Model file for the job. Use its own axes, mm. Face numbers are marked on the shaded views. A direction names the side the tool comes from. Coordinates: 2 decimals unless noted, no trailing zeros. Write each loop counter-clockwise with the first axis right and the second up, starting at its lowest first coordinate (ties: lowest second). Pieces come first, ordered by that corner, then holes. Notation, with made-up numbers: (45.25, 23.25) - (97.25, 23.25) arc R19 cw to (97.25, 55.25) - close; hole circle Ø11 at (1.25, 53.25). An arc over 180 degrees is marked (long way). Put each result on its own line as item: value. Start each with the question number.
1. Saw through at D-D, the plane z = -13. Write the cut outline in (x, y), plus the area to 3 significant figures.
2. Drop flat-ended pins along their axis: P1, Ø5, axis at y = -3.5, z = -8, coming from the -X side; P2, Ø2, axis at y = 1.5, z = -7, coming from the -X side; P3, Ø1, axis at y = 1, z = 0, coming from the -X side; P4, Ø3, axis at x = -6, z = -5, coming from the -Y side. Give the stop position or say it passes through.
3. Which spindle directions (+Z, -Z, +X, -X, +Y, -Y) get a long thin tool onto all of the face, cutting with end or side? Do the marked faces 1 and 2. Say none if no direction does.
4. Saw through at C-C, the plane x = -14.5. Write the cut outline in (y, z).
5. Drill centre lines: L1, parallel to X at y = 2, z = -10.75; L2, parallel to Z at x = -0.5, y = 2; L3, parallel to Z at x = -21, y = -1.75. Where is each one in solid material? Low to high. Write a range as from..to.
6. Saw through at A-A, the plane z = -9. Write the cut outline in (x, y), plus the area to 3 significant figures.
7. Saw through at B-B, the plane y = 0.25. Write the cut outline in (x, z).
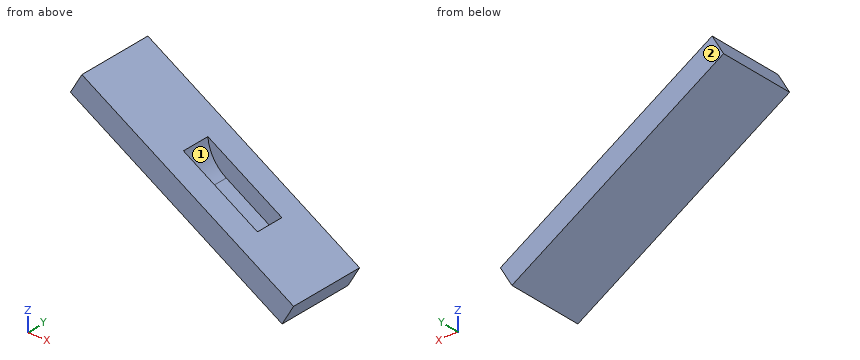
```python
from build123d import *

# Parameters (mm, degrees)
EXTRUDE_1_DEPTH      = 5
EXTRUDE_1_DEPTH_BACK = 5
CUT_EXTRUDE_1_DEPTH  = 1.85


with BuildPart() as part:
    # Sketch 2 → Extrude 1 (new body, two sides)
    with BuildSketch(Plane(origin=(0, 0, 0), x_dir=(1, 0, 0), z_dir=(0, 1, 0))) as extrude_1_sk:
        Polygon((1.795278459, 12.659996299), (-25.917534462, -3.340003701), (-27.417534462, -0.74192749), (0.295278459, 15.25807251), align=None)
    extrude(amount=EXTRUDE_1_DEPTH)
    extrude(extrude_1_sk.sketch, amount=-EXTRUDE_1_DEPTH_BACK)

    # Sketch 2_7 → Cut-Extrude 1 (cut, symmetric)
    with BuildSketch(Plane(origin=(0, 0, 0), x_dir=(1, 0, 0), z_dir=(0, 1, 0))):
        with BuildLine():
            Line((-15.35631853, -0.706584455), (-15.35631853, 2.4))
            ThreePointArc((-15.35631853, 2.4), (-14.706541739, 4.825), (-12.93131853, 6.600223208))
            Line((-12.93131853, 6.600223208), (-5.65631853, 10.800446417))
            Line((-5.65631853, 10.800446417), (-5.65631853, 4.893713156))
            Line((-5.65631853, 4.893713156), (-15.35631853, -0.706584455))
        make_face()
    extrude(amount=CUT_EXTRUDE_1_DEPTH, both=True, mode=Mode.SUBTRACT)


solid = part.part
```
Final values:
1. outline: (-3.62, -5) - (1.6, -5) - (1.6, 5) - (-3.62, 5) - close
1. area: 52.1 mm²
2. P1: stops at x = -16.61
2. P2: stops at x = -15.74
2. P3: stops at x = -27
2. P4: passes through
3. face 1: +Z, +X
3. face 2: +Z, -Z, +X, -X, +Y
4. outline: (-5, -6.72) - (5, -6.72) - (5, -3.25) - (1.85, -3.25) - (1.85, -5.15) - (-1.85, -5.15) - (-1.85, -3.25) - (-5, -3.25) - close
5. L1: x = -7.51..-1.51
5. L2: z = -14.8..-11.33
5. L3: z = -2.96..0.5
6. outline: (-10.54, -5) - (-4.54, -5) - (-4.54, 5) - (-10.54, 5) - close; hole (-8.77, -1.85) - (-5.66, -1.85) - (-5.66, 1.85) - (-8.77, 1.85) - close
6. area: 48.5 mm²
7. outline: (-27.42, 0.74) - (0.3, -15.26) - (1.8, -12.66) - (-5.66, -8.36) - (-5.66, -10.8) - (-12.93, -6.6) arc R4.85 cw to (-15.34, -2.77) - (-25.92, 3.34) - close
